from build123d import *

# Parameters (mm, degrees)
F0_W     = 38.1
F0_H     = 238.125
F1_DEPTH = 990.6
F3_DEPTH = 38.101


with BuildPart() as f1:
    # F0 (on Top) → F1 (new body)
    with BuildSketch(Plane.XY):
        with Locations((19.05, 119.0625)):
            Rectangle(F0_W, F0_H)
    extrude(amount=F1_DEPTH)

    # F2 (on face) → F3 (cut, through all)
    with BuildSketch(Plane.YZ.offset(38.1)):
        Polygon((115.270884, 0), (0, 179.310263), (-215.229422, 179.310263), (-215.229422, -479.180909), (438.821025, -479.180909), (438.821025, 1649.130165), (-444.017858, 1649.130165), (-444.017858, 591.622803), (93.90495, 937.430322), (238.125, 713.088023), (93.90495, 620.375134), (238.125, 396.032835), (93.90495, 303.319946), (238.125, 78.977646), align=None)
    extrude(amount=-F3_DEPTH, mode=Mode.SUBTRACT)


solid = f1.part
Read the model definition and answer for the solid it produces. Units are mm, in the model's axes. A direction names the side the tool comes from. Round coordinates to 2 decimals unless told otherwise and drop trailing zeros. Write each loop counter-clockwise with the first axis right and the second up, starting at its lowest first coordinate (ties: lowest second). Pieces come first, ordered by that corner, then holes.
1. The part is cut by section D-D, the plane y = 68. Determine the outline of the cut face in (x, z), then the cut area to 3 significant figures.
2. Which of the six approach directions +Z, -Z, +X, -X, +Y, -Y give full straight-line access (tool end or side, diameter ignored) to faces 1 (the face through (0, 91, 462)), 2 (the face through (19.32, 165.01, 509.77))?
3. Determine the mould class of faces 3 (the face through (19.32, 167.02, 667.38)), 4 (the face through (19, 0, 523)), 5 (the face through (19.32, 58.44, 88.4)), 6 (the face through (19.317, 46.295, 906.824)) for opening direction Z: pulls with the +Z half, pulls with the -Z half, needs draft (parallel to the pull), parting line crosses it, or undercut.
4. The part is cut by section C-C, the plane z = 98. Determine the outline of the cut face in (x, y).
5. Given pin 1 Ø6 at (x, y) = (15.5, 30.5) entering from +Z; pin 2 Ø1.5 at (x, y) = (14.5, 89.5) entering from +Z; pin 3 Ø2 at (x, y) = (7.5, 86.5) entering from +Z, each flat-ended and moving along its own axis, determine where each tip first touches the part or whether it passes through.
6. Straight lines are drawn through the part: L1, parallel to Z at x = 19.5, y = 114; L2, parallel to Z at x = 28, y = 105; L3, parallel to Z at x = 19.5, y = 74.5. For each, find the intervals that lie inside material, in ascending order.
7. The part is cut by section B-B, the plane x = 19. Determine the outline of the cut face in (y, z) (3 decimals), then the cut area to 3 significant figures.
8. The part is cut by section A-A, the plane y = 195.5. Determine the outline of the cut face in (x, z).
Values:
1. outline: (0, 73.53) - (38.1, 73.53) - (38.1, 920.78) - (0, 920.78) - close
1. area: 32,300 mm2
2. face 1: +Z, -Z, -X, +Y, -Y
2. face 2: +X, -X, +Y
3. face 3: undercut
3. face 4: needs draft
3. face 5: pulls with the -Z half
3. face 6: pulls with the +Z half
4. outline: (0, 52.27) - (38.1, 52.27) - (38.1, 225.9) - (0, 225.9) - close
5. pin 1: stops at z = 898.6
5. pin 2: stops at z = 935.08
5. pin 3: stops at z = 933.31
6. L1: z = 1.98 to 272.06, 316.24 to 589.12, 633.29 to 906.17
6. L2: z = 15.98 to 286.06, 310.45 to 603.12, 627.51 to 920.17
6. L3: z = 63.42 to 924.96
7. outline: (0, 179.31) - (115.271, 0) - (238.125, 78.978) - (93.905, 303.32) - (238.125, 396.033) - (93.905, 620.375) - (238.125, 713.088) - (93.905, 937.43) - (0, 877.063) - close
7. area: 143,000 mm2
8. outline: (0, 51.58) - (38.1, 51.58) - (38.1, 145.28) - (0, 145.28) - close; (0, 368.63) - (38.1, 368.63) - (38.1, 462.34) - (0, 462.34) - close; (0, 685.69) - (38.1, 685.69) - (38.1, 779.39) - (0, 779.39) - close
